from build123d import *

# Parameters (mm, degrees)
F0_R             = 30
F0_R_2           = 6
F1_DEPTH         = 4
F2_DEPTH         = 6
F3_W             = 3
F3_H             = 4.6
F4_DEPTH         = 9.4
F8_R             = 1.5
F9_DEPTH         = 49.2
F11_DEPTH        = 4
F11_COPIES_COUNT = 8


# Not quite as in the source:
# - a pattern or mirror of a feature is missing from the dataset's text; its kind, count and spacing are read off the source's solid


with BuildPart() as f1:
    # F0 (on Top) → F1 (new body)
    with BuildSketch(Plane.XY):
        Circle(F0_R)
        Circle(F0_R_2, mode=Mode.SUBTRACT)
        Circle(F0_R_2)
    extrude(amount=-F1_DEPTH)

    # F0 (on Top) → F2 (join)
    with BuildSketch(Plane.XY):
        Circle(F0_R_2)
    extrude(amount=F2_DEPTH)

    # F3 (on face) → F4 (cut)
    with BuildSketch(Plane.XY.offset(6)):
        with BuildLine():
            Line((1.5, -2.3), (-1.5, -2.3))
            ThreePointArc((-1.5, -2.3), (0, -2.75), (1.5, -2.3))
        make_face()
        Rectangle(F3_W, F3_H)
        with BuildLine():
            ThreePointArc((1.5, 2.3), (0, 2.75), (-1.5, 2.3))
            Line((-1.5, 2.3), (1.5, 2.3))
        make_face()
    extrude(amount=-F4_DEPTH, mode=Mode.SUBTRACT)

    # F5 (on Front) → F6 (revolve, cut)
    with BuildSketch(Plane.XZ):
        Polygon((-30, -0.5857864376), (-30, -3.4142135624), (-28.5857864376, -2), align=None)
    revolve(axis=Axis((0, 0, -0.1510307193), (0, 0, -1)), mode=Mode.SUBTRACT)

    # F8 (on offset) → F9 (cut)
    with BuildSketch(Plane.YZ.offset(25)):
        with Locations((0, 3)):
            Circle(F8_R)
    extrude(amount=-F9_DEPTH, mode=Mode.SUBTRACT)

    # F10 (on face) → F11 (cut, through all)
    with BuildSketch(Plane.XY):
        with BuildLine():
            Line((-4.2793955654, 16.3180977106), (5.1502715485, 24.0833689493))
            Line((5.1502715485, 24.0833689493), (-7.9538393766, 18.1553196162))
            ThreePointArc((-7.9538393766, 18.1553196162), (-9.040407042, 16.47119876), (-7.9538393766, 14.7870779037))
            Line((-7.9538393766, 14.7870779037), (4.9067144282, 8.9692091569))
            Line((4.9067144282, 8.9692091569), (-4.2793955654, 16.3180977106))
        make_face()
    f11 = extrude(amount=-F11_DEPTH, mode=Mode.SUBTRACT)

    # F11_copies: F11 ×8 about axis
    f11_copies_axis = Axis((0, 0, 0), (0, 0, 1))
    for i in range(1, F11_COPIES_COUNT):
        add(f11.rotate(f11_copies_axis, i * 360 / F11_COPIES_COUNT), mode=Mode.SUBTRACT)


solid = f1.part
Part model, mm, in its own coordinate system. A direction names the side the tool comes from. Give positions to 0.01 mm unless a question says otherwise; leave off trailing zeros. Use a Markdown table: item, result.
1) Two-plate mould, pull along X, no slides. Class faces 4 (the flat face through (-0.38, -12.59, -1.97)), 5 (the flat face through (0, 0, -3.4)), 6 (the flat face through (0, 0, -4)): +X half, -X half, draft (parallel to the pull), parting line (faces both ways), or undercut.
Checked values:
| item | result |
|---|---|
| face 4 | undercut |
| face 5 | undercut |
| face 6 | draft |
2) Saw through at A-A on x = 0. Count the separate pieces of the cut face and the enclosed holes in it, plus the area to 3 significant figures.
Checked values:
| item | result |
|---|---|
| separate pieces | 5 |
| enclosed holes | 0 |
| area | 227 mm² |
3) Probe L1, parallel to Z at x = -4.6, y = 0; L2, parallel to Z at x = 26, y = 3.5; L3, parallel to Y at x = -2.45, z = 3. List the from-to ranges inside material, lowest first. Write a range as from..to.
Checked values:
| item | result |
|---|---|
| L1 | -4..1.5, 4.5..6 |
| L2 | -4..0 |
| L3 | -5.48..-1.5, 1.5..5.48 |
4) 3-axis set-ups, long thin cutter, end or side, ignore diameter. For faces 1 (the cylindrical face through (-0.02, -2.75, 1.37)), 2 (the cylindrical face through (9.04, -16.5, -1.97)), 3 (the flat face through (3, 0, 6)): which of +Z, -Z, +X, -X, +Y, -Y reach the whole face in a straight line?
Checked values:
| item | result |
|---|---|
| face 1 | +Z |
| face 2 | +Z, -Z |
| face 3 | +Z, +X, -X, +Y, -Y |
5) Flat gauge pins, fed straight in: P1, Ø1.5, axis at x = 0.5, y = -0.5, coming from the +Z side; P2, Ø1, axis at x = -20.5, y = 17.5, coming from the +Z side; P3, Ø5, axis at y = 0, z = 3, coming from the -X side. Where does each tip first touch, or does it go through?
Checked values:
| item | result |
|---|---|
| P1 | z = -3.4 |
| P2 | z = 0 |
| P3 | x = -6 |
